from build123d import *

# Parameters (mm, degrees)
F0_W     = 106
F0_H     = 106
F0_W_2   = 90
F0_H_2   = 90
F1_DEPTH = 15
F2_DEPTH = 10
F3_W     = 14.440985
F3_H     = 34
F4_DEPTH = 25


with BuildPart() as f1:
    # F0 (on Front) → F1 (new body)
    with BuildSketch(Plane.XZ):
        with Locations((1.458907, 15.220348)):
            Rectangle(F0_W, F0_H)
        with Locations((1.458907, 15.220348)):
            Rectangle(F0_W_2, F0_H_2, mode=Mode.SUBTRACT)
        with Locations((1.458907, 15.220348)):
            Rectangle(F0_W_2, F0_H_2)
    extrude(amount=F1_DEPTH)

    # F0 (on Front) → F2 (cut)
    with BuildSketch(Plane.XZ):
        with Locations((1.458907, 15.220348)):
            Rectangle(F0_W, F0_H)
        with Locations((1.458907, 15.220348)):
            Rectangle(F0_W_2, F0_H_2, mode=Mode.SUBTRACT)
    extrude(amount=F2_DEPTH, mode=Mode.SUBTRACT)

    # F3 (on face) → F4 (cut)
    with BuildSketch(Plane(origin=(0, 0, 0), x_dir=(-1, 0, 0), z_dir=(0, 1, 0))):
        with Locations((-1.06852, 15.220348)):
            Rectangle(F3_W, F3_H)
    extrude(amount=-F4_DEPTH, mode=Mode.SUBTRACT)


solid = f1.part
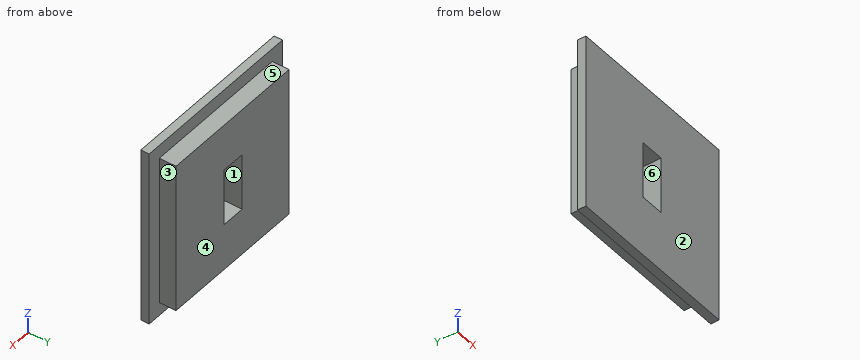
The model under review builds one solid part; all positions refer to its coordinate system, in mm. Face numbers are marked on the shaded views. A direction names the side the tool comes from. Round coordinates to 2 decimals unless told otherwise and drop trailing zeros. Order: outer loops, then holes, each group sorted by start corner. A loop starts at its lowest first (then second) coordinate and runs counter-clockwise, first axis right, second up. Notation, with made-up numbers: (13, -9.75) - (38, -9.75) arc R23 cw to (38, 5.25) - close; hole circle Ø10 at (6, 52). An arc over 180 degrees is marked (long way). Use one line per item in the form item = value.
Q1. Add section C-C on z = 28. Give the boundary of the cut face in (x, y), then the cut area to 3 significant figures.
Response values:
outline = (-51.54, -15) - (-6.15, -15) - (-6.15, 0) - (-43.54, 0) - (-43.54, -10) - (-51.54, -10) - close; (8.29, -15) - (54.46, -15) - (54.46, -10) - (46.46, -10) - (46.46, 0) - (8.29, 0) - close
area = 1,210 mm^2
Q2. Add section A-A on y = -2.25. Give the boundary of the cut face in (x, z).
Response values:
outline = (-43.54, -29.78) - (46.46, -29.78) - (46.46, 60.22) - (-43.54, 60.22) - close; hole (-6.15, -1.78) - (8.29, -1.78) - (8.29, 32.22) - (-6.15, 32.22) - close
Q3. To check wall thickness, follow line 1 (X direction, y = -4, z = 20); line 2 (X direction, y = -11.25, z = 32); line 3 (Z direction, x = 6, y = -14.5). State the ranges of each line that lie inside material, in increasing order.
Response values:
line_1 = -43.54 to -6.15, 8.29 to 46.46
line_2 = -51.54 to -6.15, 8.29 to 54.46
line_3 = -37.78 to -1.78, 32.22 to 68.22
Q4. Mouldability with a two-part tool opening along X and no side actions: class the marked faces 1, 2 and 3 as pulls with the +X half, pulls with the -X half, needs draft (parallel to the pull), parting line crosses it, or undercut.
Response values:
face_1 = undercut
face_2 = needs draft
face_3 = pulls with the +X half
Q5. Add section B-B on x = -3. Give the boundary of the cut face in (y, z), then the cut area to 3 significant figures.
Response values:
outline = (-15, -37.78) - (-10, -37.78) - (-10, -29.78) - (0, -29.78) - (0, -1.78) - (-15, -1.78) - close; (-15, 32.22) - (0, 32.22) - (0, 60.22) - (-10, 60.22) - (-10, 68.22) - (-15, 68.22) - close
area = 920 mm^2
Q6. Tool access review of the marked faces 4, 5 and 6: name each direction out of +Z, -Z, +X, -X, +Y, -Y from which nothing blocks a thin tool from reaching the whole face with its end or side.
Response values:
face_4 = +Z, -Z, +X, -X, +Y
face_5 = +Z, +X, -X, +Y
face_6 = +Y, -Y
Q7. Clearance check with flat-ended pins moving along their axes: P1, Ø5, axis at x = -1.5, y = -7, coming from the +Z side; P2, Ø3, axis at y = -3.5, z = -5, coming from the +X side; P3, Ø4, axis at y = -4, z = 40, coming from the -X side. State where each tip first meets the part, or that it passes through.
Response values:
P1 = 60.22
P2 = 46.46
P3 = -43.54
Q8. Add section D-D on x = -26.5. Give the boundary of the cut face in (y, z).
Response values:
outline = (-15, -37.78) - (-10, -37.78) - (-10, -29.78) - (0, -29.78) - (0, 60.22) - (-10, 60.22) - (-10, 68.22) - (-15, 68.22) - close
